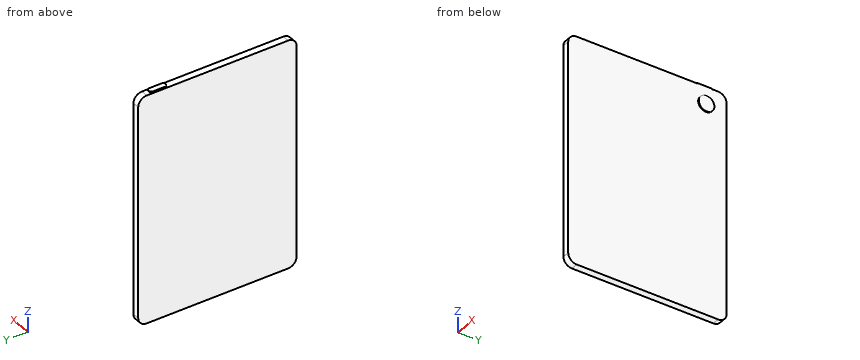
Autodesk Fusion 360 part; units mm, degrees
sketch "Sketch1" plane through (0, 0, 0) normal (1, 0, 0) x (0, 1, 0)
  line L0 (0, 0) -> (169, 0)
  line L1 (169, 0) -> (169, 242.1233)
  line L2 (169, 242.1233) -> (0, 242.1233)
  line L3 (0, 242.1233) -> (0, 0)
  dimension "d1" = 169
extrude "Extrude1" add sketch "Sketch1" along normal blind 7.5
sketch "Sketch2" plane through (0, 0, 0) normal (-1, 0, 0) x (0, -1, 0)
  line L0 (0, 0) -> (0, 242.1233)
  line L1 (0, 242.1233) -> (-169, 242.1233)
  line L2 (-169, 242.1233) -> (-169, 0)
  line L3 (-169, 0) -> (0, 0)
fillet "Fillet1" radius 9 1 edges at (3.75, 0, 242.1233)
fillet "Fillet2" radius 9 1 edges at (3.75, 169, 242.1233)
fillet "Fillet3" radius 9 1 edges at (3.75, 0, 0)
fillet "Fillet4" radius 9 1 edges at (3.75, 169, 0)
sketch "Sketch3" plane through (0, 0, 0) normal (-1, 0, 0) x (0, -1, 0)
  circle A0 centre (-85, 235) radius 5
sketch "Sketch4" plane through (0, 0, 0) normal (-1, 0, 0) x (0, -1, 0)
  circle A0 centre (-84.9515, 235.215) radius 0
sketch "Sketch5" plane through (0, 0, 0) normal (-1, 0, 0) x (0, -1, 0)
  circle A0 centre (-85.1812, 235.1149) radius 3
  dimension "d8" = 6
sketch "Sketch6" plane through (0, 0, 0) normal (-1, 0, 0) x (0, -1, 0)
  line L0 (-10, 230) -> (-160, 230)
  line L1 (-160, 230) -> (-160, 10)
  line L2 (-160, 10) -> (-10, 10)
  line L3 (-10, 10) -> (-10, 230)
sketch "Sketch7" plane through (0, 0, 0) normal (-1, 0, 0) x (0, -1, 0)
sketch "Sketch8" plane through (0, 0, 0) normal (-1, 0, 0) x (0, -1, 0)
sketch "Sketch9" plane through (0, 0, 0) normal (-1, 0, 0) x (0, -1, 0)
sketch "Sketch10" plane through (0, 0, 0) normal (-1, 0, 0) x (0, -1, 0)
sketch "Sketch11" plane through (0, 0, 0) normal (0, 0, -1) x (1, 0, 0)
  line L0 (0, -160) -> (7.5, -160)
  line L1 (7.5, -160) -> (7.5, -9)
  line L2 (7.5, -9) -> (0, -9)
  line L3 (0, -9) -> (0, -160)
sketch "Sketch12" plane through (0, 0, 242.1233) normal (0, 0, 1) x (-1, 0, 0)
  line L0 (-7.5, -160) -> (0, -160)
  line L1 (0, -160) -> (0, -9)
  line L2 (0, -9) -> (-7.5, -9)
  line L3 (-7.5, -9) -> (-7.5, -160)
  line L4 (-1, -155) -> (-7, -155)
  line L5 (-7, -155) -> (-7, -137)
  line L6 (-7, -137) -> (-1, -137)
  line L7 (-1, -137) -> (-1, -155)
extrude "Extrude2" add sketch "Sketch12" along normal blind 1 contours L4 L5 L6 L7
fillet "Fillet5" radius 2 1 edges at (1, 155, 242.6233)
fillet "Fillet6" radius 2 1 edges at (7, 155, 242.6233)
fillet "Fillet7" radius 2 1 edges at (1, 137, 242.6233)
fillet "Fillet8" radius 2 1 edges at (7, 137, 242.6233)
sketch "Sketch13" plane through (7.5, 0, 0) normal (1, 0, 0) x (0, 1, 0)
  arc A0 (160, 0) -> (169, 9) centre (160, 9) ccw
  line L0 (169, 9) -> (169, 233.1233)
  arc A1 (169, 233.1233) -> (160, 242.1233) centre (160, 233.1233) ccw
  line L1 (160, 242.1233) -> (9, 242.1233)
  arc A2 (9, 242.1233) -> (0, 233.1233) centre (9, 233.1233) ccw
  line L2 (0, 233.1233) -> (0, 9)
  arc A3 (0, 9) -> (9, 0) centre (9, 9) ccw
  line L3 (9, 0) -> (160, 0)
  circle A4 centre (146.9534, 223.7975) radius 8.2997
  circle A5 centre (147.3608, 209.8046) radius 2.0283
  dimension "d15" = 16.5995
extrude "Extrude3" add sketch "Sketch13" along normal blind 1 contours A4
CAD build for the part. Positions are in the model's coordinates, mm. Coordinates: 2 decimals unless noted, no trailing zeros. Order: outer loops, then holes, each group sorted by start corner. A loop starts at its lowest first (then second) coordinate and runs counter-clockwise, first axis right, second up. Notation, with made-up numbers: (-36.5, -5.5) -> (1.5, -5.5) arc R18 cw to (1.5, 19.5) -> close; hole circle Ø8 at (80.25, -21.75). An arc over 180 degrees is marked (long way). Use one line per item in the form item = value. Start each with the question number.
1) Drill centre lines: L1, parallel to X at y = 17.5, z = 127; L2, parallel to Z at x = 5, y = 52. Where is each one in solid material? Low to high. Write a range as [from, to].
2) Drop flat-ended pins along their axis: pin 1 (3 mm diameter, centred on y = 59.5, z = 68, fed in from +X); pin 2 (0.5 mm diameter, centred on x = 4, z = 242.5, fed in from -Y); pin 3 (1.5 mm diameter, centred on x = 2.5, y = 126, fed in from +Z). Give the stop position or say it passes through.
3) Band-saw the part on C-C on z = 20.5. Give the cut face in (x, y), then the cut area to 3 significant figures.
4) Band-saw the part on B-B on z = 226.5. Give the cut face in (x, y), then the cut area to 3 significant figures.
5) Band-saw the part on A-A on y = 148.5. Give the cut face in (x, z), then the cut area to 3 significant figures.
Entries:
q1.L1 = [0, 7.5]
q1.L2 = [0, 242.12]
q2.pin_1 = 7.5
q2.pin_2 = 137
q2.pin_3 = 242.12
q3.outline = (0, 0) -> (7.5, 0) -> (7.5, 169) -> (0, 169) -> close
q3.area = 1,270 mm2
q4.outline = (0, 0) -> (7.5, 0) -> (7.5, 139.11) -> (8.5, 139.11) -> (8.5, 154.8) -> (7.5, 154.8) -> (7.5, 169) -> (0, 169) -> close
q4.area = 1,280 mm2
q5.outline = (0, 0) -> (7.5, 0) -> (7.5, 215.64) -> (8.5, 215.64) -> (8.5, 231.95) -> (7.5, 231.95) -> (7.5, 242.12) -> (7, 242.12) -> (7, 243.12) -> (1, 243.12) -> (1, 242.12) -> (0, 242.12) -> close
q5.area = 1,840 mm2
